```python
from build123d import *

# Parameters (mm, degrees)
SKETCH1_W           = 42.0116
SKETCH1_H           = 42.0116
BOSS_EXTRUDE1_DEPTH = 48.006
CHAMFER1_SIZE       = 2.54
SKETCH2_R           = 10.9982
BOSS_EXTRUDE2_DEPTH = 1.99898
SKETCH3_R           = 2.9972
CUT_EXTRUDE1_DEPTH  = 1.016


with BuildPart() as part:
    # Sketch1 → Boss-Extrude1 (new body)
    with BuildSketch(Plane.XY):
        Rectangle(SKETCH1_W, SKETCH1_H)
    extrude(amount=BOSS_EXTRUDE1_DEPTH)

    # Chamfer1
    chamfer1_edges = [part.edges().sort_by_distance(p)[0] for p in [
        (-21.0058, 21.0058, 24.003),
        (21.0058, 21.0058, 24.003),
        (21.0058, -21.0058, 24.003),
        (-21.0058, -21.0058, 24.003),
    ]]
    chamfer(chamfer1_edges, length=CHAMFER1_SIZE)

    # Sketch2 → Boss-Extrude2 (add)
    with BuildSketch(Plane.XY.offset(48.006)):
        Circle(SKETCH2_R)
    extrude(amount=BOSS_EXTRUDE2_DEPTH)

    # Sketch3 → Cut-Extrude1 (cut)
    with BuildSketch(Plane.XY.offset(50.00498)):
        Circle(SKETCH3_R)
    extrude(amount=-CUT_EXTRUDE1_DEPTH, mode=Mode.SUBTRACT)


solid = part.part
```
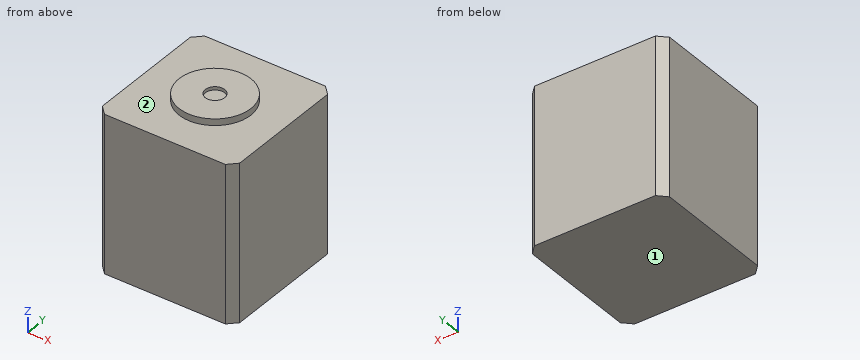
The listing builds one solid part. Answer for the finished solid, in the listing's coordinates (mm). Face numbers are marked on the shaded views. A direction names the side the tool comes from. Give positions to 0.01 mm unless a question says otherwise; leave off trailing zeros. Order: outer loops, then holes, each group sorted by start corner. A loop starts at its lowest first (then second) coordinate and runs counter-clockwise, first axis right, second up. Notation, with made-up numbers: (76, 42) -> (81, 42) arc R11 ccw to (81, 62) -> close; hole circle Ø5 at (-5, 51.5). An arc over 180 degrees is marked (long way). One line per item, written item: value.
1) A flat-ended cylindrical pin translates along its axis: P1, Ø10, axis at x = 14.5, y = -10, coming from the -Z side. Find the tip coordinate at first contact, or state that the pin passes through.
Reported:
P1: stops at z = 0
2) Find section D-D, the plane x = -17. Determine the outline of the cut face in (y, z), plus the area to 3 significant figures.
Reported:
outline: (-21.01, 0) -> (21.01, 0) -> (21.01, 48.01) -> (-21.01, 48.01) -> close
area: 2,020 mm^2
3) Find the intervals of material crossed by line 1 (Y direction, x = 0, z = 49.2); line 2 (Z direction, x = -8.5, y = -14.5), in increasing order.
Reported:
line 1: y = -11 to -3, 3 to 11
line 2: z = 0 to 48.01
4) A tool of negligible diameter and unlimited length cuts with its end or side. For the marked faces 1 and 2, from which of +Z, -Z, +X, -X, +Y, -Y can it reach the whole face along a straight path? Write none if from no direction.
Reported:
face 1: -Z, +X, -X, +Y, -Y
face 2: +Z
5) Find section C-C, the plane y = 6.5. Determine the outline of the cut face in (x, z), plus the area to 3 significant figures.
Reported:
outline: (-21.01, 0) -> (21.01, 0) -> (21.01, 48.01) -> (8.87, 48.01) -> (8.87, 50) -> (-8.87, 50) -> (-8.87, 48.01) -> (-21.01, 48.01) -> close
area: 2,050 mm^2
6) Find section A-A, the plane y = 0. Determine the outline of the cut face in (x, z), plus the area to 3 significant figures.
Reported:
outline: (-21.01, 0) -> (21.01, 0) -> (21.01, 48.01) -> (11, 48.01) -> (11, 50) -> (3, 50) -> (3, 48.99) -> (-3, 48.99) -> (-3, 50) -> (-11, 50) -> (-11, 48.01) -> (-21.01, 48.01) -> close
area: 2,050 mm^2
